Read the model definition and answer for the solid it produces. Units are mm, in the model's axes. A direction names the side the tool comes from. Give positions to 0.01 mm unless a question says otherwise; leave off trailing zeros. Loops run counter-clockwise (first coordinate to the right, second up) from the corner with the lowest first, then second, coordinate; pieces in that order, holes last.
(1) Determine the mould class of faces 6 (the face through (-43, -2.625, -7)), 7 (the face through (-17.485, 0, -20)), 8 (the face through (-41.21, -1.58, -7)), 9 (the face through (-30, 2, -15)) for opening direction Y: pulls with the +Y half, pulls with the -Y half, needs draft (parallel to the pull), parting line crosses it, or undercut.
(2) Find section A-A, the plane z = -14. Write down the section's boundary in (x, y).
(3) Straight lines are drawn through the part: probe 1 along Z at (x, y) = (-34.5, -0.65); probe 2 along X at (y, z) = (0.65, -11.5); probe 3 along Y at (x, z) = (-15, -18). For each, find the intervals that lie inside material, in ascending order.
(4) Find section B-B, the plane x = -41. Write down the section's boundary in (y, z).
(5) Which of the six approach directions +Z, -Z, +X, -X, +Y, -Y give full straight-line access (tool end or side, diameter ignored) to faces 1 (the face through (-20, 0.5, -11.257)), 2 (the face through (-37.6, 0.5, -18.257)), 3 (the face through (-33.541, -2, -7)), 4 (the face through (-44.89, 0.55, -22.22)), 5 (the face through (-28, -2, -7.757))?
(6) Find section C-C, the plane y = 0.65. State how many separate pieces and enclosed holes the cut face has, then the cut area to 3 significant figures.
(7) Each of these flat-tipped pins is pushed along its axis until it touches: P1, Ø1.6, axis at y = -2.5, z = -22, coming from the +X side; P2, Ø1.6, axis at y = 0, z = -10, coming from the -X side; P3, Ø3, axis at x = -26, z = -8, coming from the -Y side; P4, Ø10, axis at x = -18.5, z = -15, coming from the -Y side. Where does it stop, or does it pass through?
```python
from build123d import *

# Parameters (mm, degrees)
SKETCH1_W              = 22.5552
SKETCH1_H              = 12.7
BOSS_EXTRUDE1_DEPTH    = 1
SKETCH2_W              = 5
SKETCH2_H              = 7.3
CUT_EXTRUDE1_DEPTH     = 1
SKETCH3_W              = 5
SKETCH3_H              = 5
CUT_EXTRUDE2_DEPTH     = 1
BOSS_EXTRUDE2_DEPTH    = 1
SKETCH5_W              = 33.5552
SKETCH5_H              = 16.7
BOSS_EXTRUDE3_DEPTH    = 1
CUT_EXTRUDE4_DEPTH     = 1
CUT_EXTRUDE5_START     = -4
CUT_EXTRUDE5_DEPTH     = 5
SKETCH10_W             = 22.5552
SKETCH10_H             = 2
BOSS_EXTRUDE4_DEPTH    = 2
SKETCH11_W             = 8.919893548
SKETCH11_H             = 0.730490532
CUT_EXTRUDE6_DEPTH     = 3
SKETCH12_W             = 22.5552
SKETCH12_H             = 1.5
BOSS_EXTRUDE5_DEPTH    = 2
SKETCH13_W             = 3
SKETCH13_H             = 1.5
CUT_EXTRUDE7_DEPTH     = 2
SKETCH14_W             = 2.125
SKETCH14_H             = 1.226869322
CUT_EXTRUDE8_DEPTH     = 1
SKETCH15_W             = 2.12
SKETCH15_H             = 12
ADAPTER_PCB_HOLE_DEPTH = 1
SKETCH16_W             = 7
SKETCH16_H             = 1.5
BOSS_EXTRUDE6_DEPTH    = 4
NUT_HOLE_DEPTH         = 1.5
SKETCH20_W             = 7
SKETCH20_H             = 1.5
BOSS_EXTRUDE7_DEPTH    = 4
NUT_HOLE2_DEPTH        = 1.5


with BuildPart() as part:
    # Sketch1 → Boss-Extrude1 (new body)
    with BuildSketch(Plane(origin=(0, 0, 0), x_dir=(1, 0, 0), z_dir=(0, 1, 0))):
        with Locations((-28.763088774, 14.606547542)):
            Rectangle(SKETCH1_W, SKETCH1_H)
    extrude(amount=BOSS_EXTRUDE1_DEPTH)

    # Sketch2 → Cut-Extrude1 (cut)
    with BuildSketch(Plane(origin=(0, 1, 0), x_dir=(1, 0, 0), z_dir=(0, 1, 0))):
        with Locations((-37.540688774, 14.606547542)):
            Rectangle(SKETCH2_W, SKETCH2_H)
    extrude(amount=-CUT_EXTRUDE1_DEPTH, mode=Mode.SUBTRACT)

    # Sketch3 → Cut-Extrude2 (cut)
    with BuildSketch(Plane(origin=(0, 1, 0), x_dir=(1, 0, 0), z_dir=(0, 1, 0))):
        with Locations((-19.985488774, 13.756547542)):
            Rectangle(SKETCH3_W, SKETCH3_H)
    extrude(amount=-CUT_EXTRUDE2_DEPTH, mode=Mode.SUBTRACT)

    # Sketch4 → Boss-Extrude2 (add)
    with BuildSketch(Plane.XZ):
        Polygon((-40.040688774, -8.256547542), (-40.040688774, -8.756547542), (-17.985488774, -8.756547542), (-17.985488774, -10.256547542), (-17.485488774, -10.256547542), (-17.485488774, -8.256547542), align=None)
        Polygon((-17.985488774, -20.456547542), (-40.040688774, -20.456547542), (-40.040688774, -20.956547542), (-17.485488774, -20.956547542), (-17.485488774, -18.456547542), (-17.985488774, -18.456547542), align=None)
    extrude(amount=BOSS_EXTRUDE2_DEPTH)

    # Sketch5 → Boss-Extrude3 (add)
    with BuildSketch(Plane(origin=(0, 1, 0), x_dir=(1, 0, 0), z_dir=(0, 1, 0))):
        with Locations((-30.263088774, 14.606547542)):
            Rectangle(SKETCH5_W, SKETCH5_H)
    extrude(amount=BOSS_EXTRUDE3_DEPTH)

    # Sketch7 → Cut-Extrude4 (cut)
    with BuildSketch(Plane(origin=(0, 1, 0), x_dir=(-1, 0, 0), z_dir=(0, -1, 0))):
        Polygon((17.735488774, 14.983416864), (15.610488774, 16.210286186), (13.485488774, 14.983416864), (13.485488774, 12.52967822), (15.610488774, 11.302808898), (17.735488774, 12.52967822), align=None)
    extrude(amount=-CUT_EXTRUDE4_DEPTH, mode=Mode.SUBTRACT)

    # Sketch8 → Cut-Extrude5 (cut)
    with BuildSketch(Plane(origin=(0, 2, 0), x_dir=(1, 0, 0), z_dir=(0, 1, 0)).offset(CUT_EXTRUDE5_START)):
        with BuildLine():
            Line((-13.485488774, 22.956547542), (-22.127760886, 22.956547542))
            add(Edge.make_bspline(
                [(-22.127760886, 22.956547542), (-17.367981555, 22.956547542), (-14.30272025, 21.87197064), (-13.485488774, 18.176213027)],
                knots=[0, 0, 0, 0, 1, 1, 1, 1], degree=3))
            Line((-13.485488774, 18.176213027), (-13.485488774, 22.956547542))
        make_face()
    cut_extrude5 = extrude(amount=CUT_EXTRUDE5_DEPTH, mode=Mode.SUBTRACT)

    # Mirror2: Cut-Extrude5 across plane
    add(cut_extrude5.mirror(Plane.XY.offset(-14.61)), mode=Mode.SUBTRACT)

    # Sketch10 → Boss-Extrude4 (add)
    with BuildSketch(Plane(origin=(0, 1, 0), x_dir=(-1, 0, 0), z_dir=(0, -1, 0))):
        with Locations((28.763088774, 7.256547542)):
            Rectangle(SKETCH10_W, SKETCH10_H)
        with Locations((28.763088774, 21.956547542)):
            Rectangle(SKETCH10_W, SKETCH10_H)
    extrude(amount=BOSS_EXTRUDE4_DEPTH)

    # Sketch11 → Cut-Extrude6 (cut)
    with BuildSketch(Plane(origin=(0, 2, 0), x_dir=(1, 0, 0), z_dir=(0, 1, 0))):
        with Locations((-17.667814112, 5.898207192)):
            Rectangle(SKETCH11_W, SKETCH11_H)
    extrude(amount=-CUT_EXTRUDE6_DEPTH, mode=Mode.SUBTRACT)

    # Sketch12 → Boss-Extrude5 (add)
    with BuildSketch(Plane(origin=(0, -1, 0), x_dir=(-1, 0, 0), z_dir=(0, -1, 0))):
        with Locations((28.763088774, 7.006547542)):
            Rectangle(SKETCH12_W, SKETCH12_H)
        with Locations((28.763088774, 22.206547542)):
            Rectangle(SKETCH12_W, SKETCH12_H)
    extrude(amount=BOSS_EXTRUDE5_DEPTH)

    # Sketch13 → Cut-Extrude7 (cut)
    with BuildSketch(Plane(origin=(0, -3, 0), x_dir=(-1, 0, 0), z_dir=(0, -1, 0))):
        with Locations((35.040688774, 7.006547542)):
            Rectangle(SKETCH13_W, SKETCH13_H)
        with Locations((35.040688774, 22.206547542)):
            Rectangle(SKETCH13_W, SKETCH13_H)
        with Locations((22.040688774, 7.006547542)):
            Rectangle(SKETCH13_W, SKETCH13_H)
        with Locations((22.040688774, 22.206547542)):
            Rectangle(SKETCH13_W, SKETCH13_H)
    extrude(amount=-CUT_EXTRUDE7_DEPTH, mode=Mode.SUBTRACT)

    # Sketch14 → Cut-Extrude8 (cut)
    with BuildSketch(Plane(origin=(0, 2, 0), x_dir=(1, 0, 0), z_dir=(0, 1, 0))):
        with Locations((-14.547988774, 15.596851525)):
            Rectangle(SKETCH14_W, SKETCH14_H)
        with Locations((-14.547988774, 11.916243559)):
            Rectangle(SKETCH14_W, SKETCH14_H)
    extrude(amount=-CUT_EXTRUDE8_DEPTH, mode=Mode.SUBTRACT)

    # Sketch15 → adapter_PCB_hole (cut)
    with BuildSketch(Plane(origin=(0, 1, 0), x_dir=(-1, 0, 0), z_dir=(0, -1, 0))):
        with Locations((45.100688774, 14.606547542)):
            Rectangle(SKETCH15_W, SKETCH15_H)
    extrude(amount=-ADAPTER_PCB_HOLE_DEPTH, mode=Mode.SUBTRACT)

    # Sketch16 → Boss-Extrude6 (add)
    with BuildSketch(Plane(origin=(0, 1, 0), x_dir=(-1, 0, 0), z_dir=(0, -1, 0))):
        with Locations((43.540688774, 22.206547542)):
            Rectangle(SKETCH16_W, SKETCH16_H)
    extrude(amount=BOSS_EXTRUDE6_DEPTH)

    # Sketch19 → nut_hole (cut)
    with BuildSketch(Plane(origin=(0, 0, -22.956547542), x_dir=(-1, 0, 0), z_dir=(0, 0, -1))):
        Polygon((45.494427418, -0.5), (44.267558096, 1.625), (41.813819452, 1.625), (40.58695013, -0.5), (41.813819452, -2.625), (44.267558096, -2.625), align=None)
    extrude(amount=-NUT_HOLE_DEPTH, mode=Mode.SUBTRACT)

    # Sketch20 → Boss-Extrude7 (add)
    with BuildSketch(Plane(origin=(0, 1, 0), x_dir=(-1, 0, 0), z_dir=(0, -1, 0))):
        with Locations((43.540688774, 7.006547542)):
            Rectangle(SKETCH20_W, SKETCH20_H)
    extrude(amount=BOSS_EXTRUDE7_DEPTH)

    # Sketch21 → nut_hole2 (cut)
    with BuildSketch(Plane.XY.offset(-6.256547542)):
        Polygon((-45.494427418, -0.5), (-44.267558096, -2.625), (-41.813819452, -2.625), (-40.58695013, -0.5), (-41.813819452, 1.625), (-44.267558096, 1.625), align=None)
    extrude(amount=-NUT_HOLE2_DEPTH, mode=Mode.SUBTRACT)


solid = part.part
```
Entries:
1. face 6: undercut
1. face 7: needs draft
1. face 8: undercut
1. face 9: pulls with the +Y half
2. outline: (-47.04, 1) - (-46.16, 1) - (-46.16, 2) - (-47.04, 2) - close; (-44.04, 1) - (-35.04, 1) - (-35.04, 0) - (-22.49, 0) - (-22.49, 1) - (-17.74, 1) - (-17.74, 2) - (-44.04, 2) - close
3. probe 1: z = -22.96 to -20.46, -8.76 to -6.26
3. probe 2: x = -35.04 to -22.49
3. probe 3: y = 1 to 2
4. outline: (-3, -22.96) - (-1.22, -22.96) - (-1.22, -21.46) - (-3, -21.46) - close; (-3, -7.76) - (-1.22, -7.76) - (-1.22, -6.26) - (-3, -6.26) - close; (0.22, -22.96) - (2, -22.96) - (2, -6.26) - (0.22, -6.26) - (0.22, -7.76) - (1, -7.76) - (1, -21.46) - (0.22, -21.46) - close
5. face 1: +X, -Y
5. face 2: -X, -Y
5. face 3: +Z, -Z, -Y
5. face 4: -Z
5. face 5: +X, -X, -Y
6. separate pieces: 3
6. enclosed holes: 0
6. area: 325 mm2
7. P1: stops at x = -17.49
7. P2: stops at x = -40.04
7. P3: stops at y = -3
7. P4: stops at y = -1
